```python
from build123d import *

# Parameters (mm, degrees)
SKETCH1_R           = 30.5943
BOSS_EXTRUDE1_DEPTH = 38.1
SHELL1_T            = -0.254
FILLET1_R           = 2.54
FILLET2_R           = 2.54


with BuildPart() as part:
    # Sketch1 → Boss-Extrude1 (new body)
    with BuildSketch(Plane(origin=(0, 0, 0), x_dir=(1, 0, 0), z_dir=(0, 1, 0))):
        with Locations(Location((0, 0, 0), (0, 0, 90))):
            Circle(SKETCH1_R)
    extrude(amount=BOSS_EXTRUDE1_DEPTH)

    # Shell1
    shell1_openings = [part.faces().sort_by_distance(p)[0] for p in [
        (0, 0, 0),
    ]]
    offset(amount=SHELL1_T, openings=shell1_openings, kind=Kind.INTERSECTION)

    # Fillet1
    fillet1_edges = [part.edges().sort_by_distance(p)[0] for p in [
        (0, 37.846, 30.3403),
    ]]
    fillet(fillet1_edges, radius=FILLET1_R)

    # Fillet2
    fillet2_edges = [part.edges().sort_by_distance(p)[0] for p in [
        (0, 38.1, 30.5943),
    ]]
    fillet(fillet2_edges, radius=FILLET2_R)


solid = part.part
```
Can you work these out from the model? Positions are in its coordinate system, mm. Coordinates: 2 decimals unless noted, no trailing zeros. Loops run counter-clockwise (first coordinate to the right, second up) from the corner with the lowest first, then second, coordinate; pieces in that order, holes last.
1) Thinking about a two-plate mould opening in X: for faces 1 (the flat face through (0, 38.1, 0)), 2 (the cylindrical face through (-30.334, 17.531, 3.983)), 3 (the cylindrical face through (29.62, 17.41, 6.58)), which applies, pulls with the +X half, pulls with the -X half, needs draft (parallel to the pull), parting line crosses it, or undercut?
2) Imagine slicing it at C-C on y = 8. List the corners of the cut face in (x, z) for me, plus the area to 3 significant figures.
3) Imagine slicing it at A-A on z = 0. List the corners of the cut face in (x, y) for me.
4) I need wall thicknesses on probe 1 along X at (y, z) = (16, 0); probe 2 along Y at (x, z) = (-15, -9); probe 3 along X at (y, z) = (15, 20.5). Which ranges of each line are inside material? Lowest first, please.
5) For pin 1 (4 mm diameter, centred on y = 14.5, z = 4, fed in from -X); pin 2 (16.5 mm diameter, centred on x = -0.5, z = -4, fed in from -Y); pin 3 (12 mm diameter, centred on y = 17, z = 22, fed in from +X), each with a flat end and sliding along its axis, tell me the tip position at first contact or that it passes through.
6) Imagine slicing it at B-B on x = 0. List the corners of the cut face in (y, z) for me, plus the area to 3 significant figures.
Completed:
1. face 1: needs draft
1. face 2: parting line crosses it
1. face 3: undercut
2. outline: circle Ø61.19 at (0, 0); hole circle Ø60.68 at (0, 0)
2. area: 48.6 mm2
3. outline: (-30.59, 0) - (-30.34, 0) - (-30.34, 35.31) arc R2.54 cw to (-27.8, 37.85) - (27.8, 37.85) arc R2.54 cw to (30.34, 35.31) - (30.34, 0) - (30.59, 0) - (30.59, 35.56) arc R2.54 ccw to (28.05, 38.1) - (-28.05, 38.1) arc R2.54 ccw to (-30.59, 35.56) - close
4. probe 1: x = -30.59 to -30.34, 30.34 to 30.59
4. probe 2: y = 37.85 to 38.1
4. probe 3: x = -22.71 to -22.37, 22.37 to 22.71
5. pin 1: stops at x = -30.53
5. pin 2: stops at y = 37.85
5. pin 3: stops at x = 26.08
6. outline: (0, -30.59) - (35.56, -30.59) arc R2.54 ccw to (38.1, -28.05) - (38.1, 28.05) arc R2.54 ccw to (35.56, 30.59) - (0, 30.59) - (0, 30.34) - (35.31, 30.34) arc R2.54 cw to (37.85, 27.8) - (37.85, -27.8) arc R2.54 cw to (35.31, -30.34) - (0, -30.34) - close
6. area: 34.8 mm2
